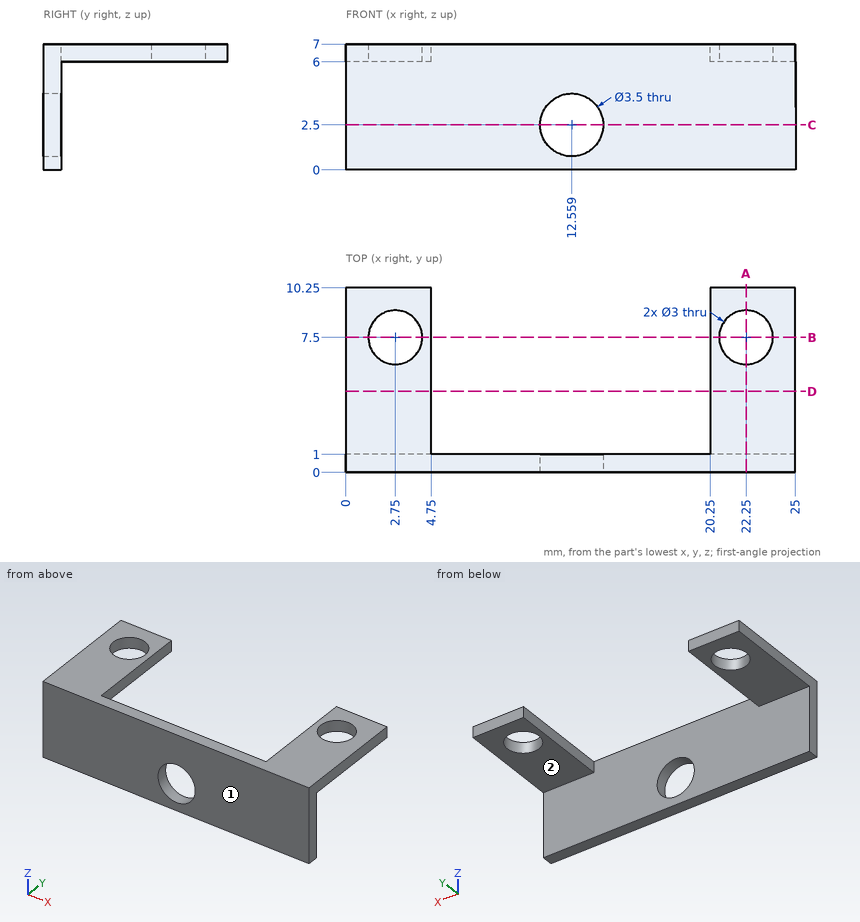
Source: three-view drawing plus pictorial views. Frame: mm from the lowest corner of the part. A direction names the side the tool comes from. Coordinates: 2 decimals unless noted, no trailing zeros. Loops run counter-clockwise (first coordinate to the right, second up) from the corner with the lowest first, then second, coordinate; pieces in that order, holes last. Notation, with made-up numbers: (-26, 38.5) -> (19, 38.5) arc R18 ccw to (19, 73.5) -> close; hole circle Ø10 at (65.5, 47). An arc over 180 degrees is marked (long way). Answer in a Markdown table with one row per item. Add a question column.
Q1. Section D-D on y = 4.5. Return the cut outline in (x, z).
Q2. Section C-C on z = 2.5. Return the cut outline in (x, y).
Q3. Contact query for flat-ended pins moving along their axis: pin 1 Ø3.5 at (x, z) = (9.5, 2.5) entering from +Y; pin 2 Ø5 at (x, y) = (2.5, 7.5) entering from -Z. Output: stop coordinate, or through.
Q4. Section B-B on y = 7.5. Return the cut outline in (x, z).
Q5. Section A-A on x = 22.25. Return the cut outline in (y, z).
Q6. Ray query, line 1 along Y through (x, z) = (2.75, 6.3); line 2 along X through (y, z) = (0.5, 2.5); line 3 along Y through (x, z) = (8.75, 0.5). Return the intervals inside material, ascending.
Q7. Reachability of the marked faces 1 and 2 from +Z, -Z, +X, -X, +Y, -Y: full face, straight path, thin tool, end or side. Return the list, or none.
Computed values:
| question | item | result |
|---|---|---|
| 1 | outline | (0, 6) -> (4.75, 6) -> (4.75, 7) -> (0, 7) -> close; (20.25, 6) -> (25, 6) -> (25, 7) -> (20.25, 7) -> close |
| 2 | outline | (0, 0) -> (10.81, 0) -> (10.81, 1) -> (0, 1) -> close; (14.31, 0) -> (25, 0) -> (25, 1) -> (14.31, 1) -> close |
| 3 | pin 1 | stops at y = 1 |
| 3 | pin 2 | stops at z = 6 |
| 4 | outline | (0, 6) -> (1.25, 6) -> (1.25, 7) -> (0, 7) -> close; (4.25, 6) -> (4.75, 6) -> (4.75, 7) -> (4.25, 7) -> close; (20.25, 6) -> (20.75, 6) -> (20.75, 7) -> (20.25, 7) -> close; (23.75, 6) -> (25, 6) -> (25, 7) -> (23.75, 7) -> close |
| 5 | outline | (0, 0) -> (1, 0) -> (1, 6) -> (6, 6) -> (6, 7) -> (0, 7) -> close; (9, 6) -> (10.25, 6) -> (10.25, 7) -> (9, 7) -> close |
| 6 | line 1 | y = 0 to 6, 9 to 10.25 |
| 6 | line 2 | x = 0 to 10.81, 14.31 to 25 |
| 6 | line 3 | y = 0 to 1 |
| 7 | face 1 | +Z, -Z, +X, -X, -Y |
| 7 | face 2 | -Z, +X, -X, +Y |
